```python
from build123d import *

# Parameters (mm, degrees)
SKETCH2_R           = 1
BOSS_EXTRUDE1_DEPTH = 1
BOSS_EXTRUDE2_START = 2.5
SKETCH2_3_R         = 1.5
SKETCH2_3_R_2       = 1
BOSS_EXTRUDE2_DEPTH = 2.5


with BuildPart() as part:
    # Sketch2 → Boss-Extrude1 (new body)
    with BuildSketch(Plane.YZ):
        with BuildLine():
            ThreePointArc((-2.777777778, 3.362258757), (-7.25, 0), (-2.777777778, -3.362258757))
            ThreePointArc((-2.777777778, -3.362258757), (0, -2.968712349), (2.777777778, -3.362258757))
            ThreePointArc((2.777777778, -3.362258757), (7.25, 0), (2.777777778, 3.362258757))
            ThreePointArc((2.777777778, 3.362258757), (0, 2.968712349), (-2.777777778, 3.362258757))
        make_face()
        with Locations(Location((-3.75, 0, 0), (0, 0, 270))):
            Circle(SKETCH2_R, mode=Mode.SUBTRACT)
        with Locations(Location((3.75, 0, 0), (0, 0, 270))):
            Circle(SKETCH2_R, mode=Mode.SUBTRACT)
    extrude(amount=-BOSS_EXTRUDE1_DEPTH)

    # Sketch2_3 → Boss-Extrude2 (add)
    # profile 1 of 2: a face of its own
    with BuildSketch(Plane.YZ.offset(BOSS_EXTRUDE2_START)):
        with Locations(Location((-3.75, 0, 0), (0, 0, 270))):
            Circle(SKETCH2_3_R)
        with Locations(Location((-3.75, 0, 0), (0, 0, 270))):
            Circle(SKETCH2_3_R_2, mode=Mode.SUBTRACT)
    # profile 2 of 2: a face of its own
    with BuildSketch(Plane.YZ.offset(BOSS_EXTRUDE2_START)):
        with Locations(Location((3.75, 0, 0), (0, 0, 270))):
            Circle(SKETCH2_3_R)
        with Locations(Location((3.75, 0, 0), (0, 0, 270))):
            Circle(SKETCH2_3_R_2, mode=Mode.SUBTRACT)
    extrude(amount=-BOSS_EXTRUDE2_DEPTH)

    # Mirror1: part across plane


with BuildPart() as part_1:
    add(part.part)
    add(part.part.mirror(Plane(origin=(2.5, 0, 0), x_dir=(0, 0, 1), z_dir=(1, 0, 0))))


solid = part_1.part
```
Source: CAD feature listing. Evaluate the final solid. Frame: model axes, mm. A direction names the side the tool comes from. Coordinates: 2 decimals unless noted, no trailing zeros. Loops run counter-clockwise (first coordinate to the right, second up) from the corner with the lowest first, then second, coordinate; pieces in that order, holes last. Notation, with made-up numbers: (17.25, 36) -> (49.25, 36) arc R33 ccw to (49.25, 68) -> close; hole circle Ø10 at (46.25, 63.25). An arc over 180 degrees is marked (long way). One line per item, written item: value. Start each with the question number.
Q1. Section query B-B, the plane y = -3.75. Return the cut outline in (x, z).
Q2. Set-up query: faces 3 (the face through (-1, 0, 0)), 4 (the face through (5, 0, 0)). Return all of +Z, -Z, +X, -X, +Y, -Y with unobstructed straight access to the full face (end or side cutting, diameter ignored); none if empty.
Q3. Contact query for flat-ended pins moving along their axis: P1, Ø4, axis at x = 5, y = 0.5, coming from the -Z side; P2, Ø1.8, axis at y = -3.75, z = 0, coming from the -X side. Output: stop coordinate, or through.
Q4. Mould query, pull axis Y, two halves, no side actions, for faces 1 (the face through (6, 0, 0)), 2 (the face through (-0.49, 0.04, 2.97)). Classes: pulls with the +Y half, pulls with the -Y half, needs draft (parallel to the pull), parting line crosses it, or undercut.
Q5. Section query D-D, the plane z = -2.5. Return the cut outline in (x, y).
Q6. Section query A-A, the plane z = 0. Return the cut outline in (x, y), and give its area (3 significant figures).
Q7. Section query C-C, the plane x = 0.5. Return the cut outline in (y, z).
Q8. Line query: line 1 along Y through (x, z) = (3, 0); line 2 along X through (y, z) = (-1.25, -0.75); line 3 along Y through (x, z) = (5.75, 0.75). Output: solid intervals per line, ascending.
Results:
1. outline: (-1, -3.5) -> (0, -3.5) -> (0, -1.5) -> (5, -1.5) -> (5, -3.5) -> (6, -3.5) -> (6, -1) -> (-1, -1) -> close; (-1, 1) -> (6, 1) -> (6, 3.5) -> (5, 3.5) -> (5, 1.5) -> (0, 1.5) -> (0, 3.5) -> (-1, 3.5) -> close
2. face 3: +Z, -Z, -X, +Y, -Y
2. face 4: none
3. P1: z = -3.29
3. P2: through
4. face 1: needs draft
4. face 2: undercut
5. outline: (-1, -6.2) -> (0, -6.2) -> (0, 6.2) -> (-1, 6.2) -> close; (5, -6.2) -> (6, -6.2) -> (6, 6.2) -> (5, 6.2) -> close
6. outline: (-1, -7.25) -> (0, -7.25) -> (0, -5.25) -> (5, -5.25) -> (5, -7.25) -> (6, -7.25) -> (6, -4.75) -> (-1, -4.75) -> close; (-1, -2.75) -> (6, -2.75) -> (6, 2.75) -> (-1, 2.75) -> close; (-1, 4.75) -> (6, 4.75) -> (6, 7.25) -> (5, 7.25) -> (5, 5.25) -> (0, 5.25) -> (0, 7.25) -> (-1, 7.25) -> close; hole (0, -2.25) -> (5, -2.25) -> (5, 2.25) -> (0, 2.25) -> close
6. area: 31.0 mm^2
7. outline: circle Ø3 at (-3.75, 0); circle Ø3 at (3.75, 0); hole circle Ø2 at (-3.75, 0); hole circle Ø2 at (3.75, 0)
8. line 1: -5.25 to -4.75, -2.75 to -2.25, 2.25 to 2.75, 4.75 to 5.25
8. line 2: -1 to 0, 5 to 6
8. line 3: -7.17 to -4.41, -3.09 to 3.09, 4.41 to 7.17
